Input: dimensioned drawing with shaded views. Units: mm. Origin: part minimum x, y, z. A direction names the side the tool comes from. Give positions to 0.01 mm unless a question says otherwise; leave off trailing zeros. Order: outer loops, then holes, each group sorted by start corner. A loop starts at its lowest first (then second) coordinate and runs counter-clockwise, first axis right, second up. Notation, with made-up numbers: (51.25, -22.5) -> (66.25, -22.5) arc R31 ccw to (66.25, 7.5) -> close; hole circle Ø6 at (-37.75, -6). An arc over 180 degrees is marked (long way). Use CSV: the item, a comma, the result in double quotes.
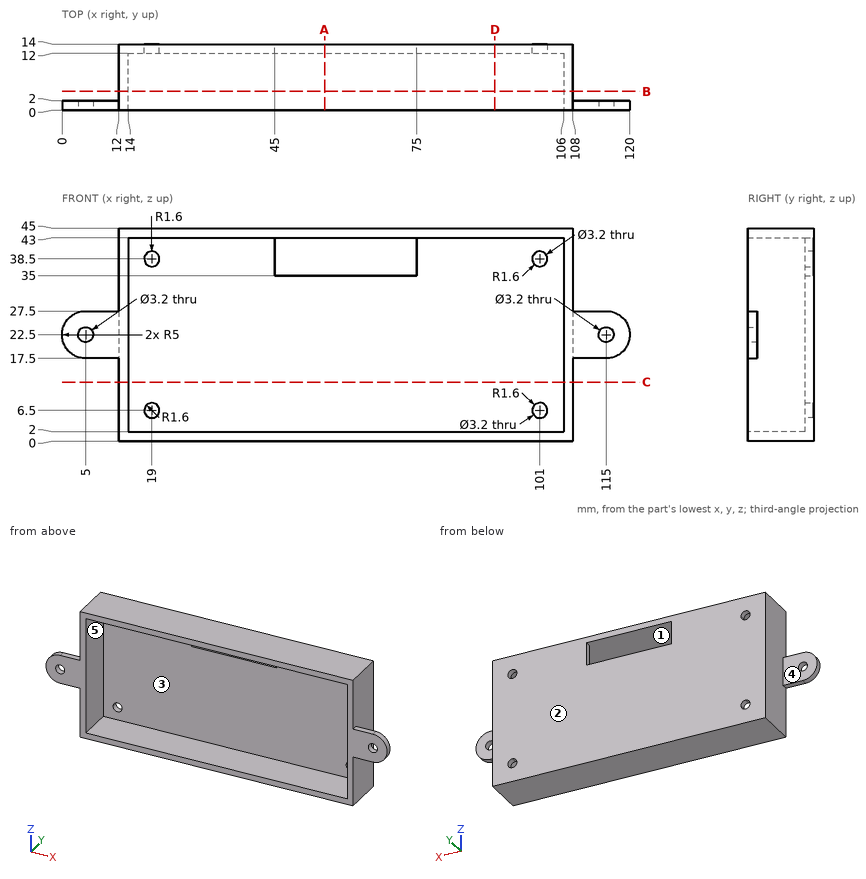
1. Section query B-B on y = 4. Return loops of the section in (x, z).
Answer below:
outline,"(12, 0) -> (108, 0) -> (108, 45) -> (12, 45) -> close; hole (14, 2) -> (106, 2) -> (106, 43) -> (14, 43) -> close"
2. Ray query, line 1 along X through (y, z) = (1.05, 22.5); line 2 along Z through (x, y) = (101, 12.9); line 3 along X through (y, z) = (12.65, 6.5). Return the intervals inside material, ascending.
Answer below:
line 1,"x = 0 to 3.4, 6.6 to 14, 106 to 113.4, 116.6 to 120"
line 2,"z = 0 to 4.9, 8.1 to 36.9, 40.1 to 45"
line 3,"x = 12 to 17.4, 20.6 to 99.4, 102.6 to 108"
3. Mould query, pull axis X, two halves, no side actions, for the marked faces 3, 4 and 5. Classes: released by +X, released by -X, zero draft, split by the parting line, or undercut.
Answer below:
face 3,"undercut"
face 4,"zero draft"
face 5,"undercut"
4. Pin query (flat end, axial travel): P1, Ø3, axis at x = 7, z = 23.5, coming from the +Y side; P2, Ø1, axis at x = 8.5, y = 1, coming from the +Z side; P3, Ø12.5, axis at x = 42.5, z = 17, coming from the -Y side. Return the tip coordinate at first contact, or that it passes through.
Answer below:
P1,"stops at y = 2"
P2,"stops at z = 27.5"
P3,"stops at y = 12"
5. Section query D-D on x = 91.5. Return loops of the section in (y, z), plus the area to 3 significant figures.
Answer below:
outline,"(0, 0) -> (14, 0) -> (14, 45) -> (0, 45) -> (0, 43) -> (12, 43) -> (12, 2) -> (0, 2) -> close"
area,"138 mm²"
6. Section query C-C on z = 12.5. Return loops of the section in (x, y), plus the area to 3 significant figures.
Answer below:
outline,"(12, 0) -> (14, 0) -> (14, 12) -> (106, 12) -> (106, 0) -> (108, 0) -> (108, 14) -> (12, 14) -> close"
area,"240 mm²"
7. Access query for the marked faces 1 and 2. Directions: +Z, -Z, +X, -X, +Y, -Y. A direction counts if a zero-diameter tool reaches every point of the face in a straight line with its end or side. Return the directions, or none.
Answer below:
face 1,"-Y"
face 2,"+Z, -Z, +X, -X, +Y"
8. Section query A-A on x = 55.5. Return loops of the section in (y, z).
Answer below:
outline,"(0, 0) -> (14, 0) -> (14, 35) -> (12, 35) -> (12, 2) -> (0, 2) -> close; (0, 43) -> (14, 43) -> (14, 45) -> (0, 45) -> close"
